```python
from build123d import *

# Parameters (mm, degrees)
SALIENTE_EXTRUIR1_DEPTH      = 6.5
SALIENTE_EXTRUIR1_DEPTH_BACK = 30
CROQUIS1_R                   = 2
CROQUIS2_W                   = 8
CROQUIS2_H                   = 10
CROQUIS2_H_2                 = 17.5
CORTAR_EXTRUIR2_DEPTH        = 20


with BuildPart() as part:
    # Croquis1 → Saliente-Extruir1 (new, two sides: drawn at the far end of the back side and taken through both)
    with BuildSketch(Plane.XY.offset(-SALIENTE_EXTRUIR1_DEPTH_BACK)):
        with BuildLine():
            Line((28.793175074, 33.764978898), (7.779852304, 40.592621349))
            Line((7.779852304, 40.592621349), (6.543784327, 36.788395284))
            ThreePointArc((6.543784327, 36.788395284), (4.366334456, 31.125676473), (9.776753104, 33.870679629))
            ThreePointArc((9.776753104, 33.870679629), (16.738586943, 32.414771462), (23.226590181, 29.500562652))
            ThreePointArc((23.226590181, 29.500562652), (25.990238441, 24.099644159), (27.557107096, 29.960752833))
            Line((27.557107096, 29.960752833), (28.793175074, 33.764978898))
        make_face()
        with Locations((6.543784327, 33.538395284)):
            Circle(CROQUIS1_R, mode=Mode.SUBTRACT)
        with Locations((25.646805026, 27.331447601)):
            Circle(CROQUIS1_R, mode=Mode.SUBTRACT)
    extrude(amount=SALIENTE_EXTRUIR1_DEPTH + SALIENTE_EXTRUIR1_DEPTH_BACK)

    # Croquis2 → Cortar-Extruir2 (cut)
    with BuildSketch(Plane(origin=(12.672781879, 39.002812158, 0), x_dir=(0.9510565162951536, -0.3090169943749473, 0), z_dir=(0.3090169943749473, 0.9510565162951536, 0))):
        with Locations((-3.390425382, 25)):
            Rectangle(CROQUIS2_W, CROQUIS2_H)
        with Locations((-3.390425382, -1.5)):
            Rectangle(CROQUIS2_W, CROQUIS2_H)
        with Locations((15.195679253, 11.75)):
            Rectangle(CROQUIS2_W, CROQUIS2_H_2)
    extrude(amount=-CORTAR_EXTRUIR2_DEPTH, mode=Mode.SUBTRACT)


solid = part.part
```
Part model, mm, in its own coordinate system. A direction names the side the tool comes from. Coordinates: 2 decimals unless noted, no trailing zeros. Order: outer loops, then holes, each group sorted by start corner. A loop starts at its lowest first (then second) coordinate and runs counter-clockwise, first axis right, second up. Notation, with made-up numbers: (-26, 39.25) -> (-1, 39.25) arc R25 cw to (-1, 67.25) -> close; hole circle Ø9 at (48.5, -0.5). An arc over 180 degrees is marked (long way). Put each result on its own line as item: value. Start each with the question number.
(1) Mould opens along Y. For faces 5 (the face through (12.424, 36.265, -24.93)), 6 (the face through (28.166, 31.836, 1.683)), 7 (the face through (26, 31, -20.5)) say: pulls with the +Y half, pulls with the -Y half, needs draft (parallel to the pull), parting line crosses it, or undercut.
(2) Band-saw the part on A-A (y = 26.5). Give the cut face in (x, z).
(3) Band-saw the part on C-C (y = 31). Give the cut face in (x, z).
(4) Band-saw the part on D-D (z = -8.5). Give the cut face in (x, y).
(5) Probe line 1 along Z through (x, y) = (27.5, 31.5); line 2 along X through (y, z) = (26, -2.5); line 3 along Z through (x, y) = (10.75, 39). List the from-to ranges inside material, lowest first. Write a range as [from, to].
(6) Which spindle directions (+Z, -Z, +X, -X, +Y, -Y) get a long thin tool onto all of the face, cutting with end or side? Do faces 1 (the face through (12.424, 36.265, 1.57)), 2 (the face through (28.166, 31.836, -25.316)), 3 (the face through (22.49, 32.99, -11.63)), 4 (the face through (22, 33, 6.5)). Say none if no direction does.
(7) Pin check, flat tips, straight feed: pin 1 Ø1.5 at (y, z) = (39, -2.5) entering from -X; pin 2 Ø5 at (x, y) = (8, 36.5) entering from +Z; pin 3 Ø3.5 at (x, y) = (25.65, 27.33) entering from -Z; pin 4 Ø10 at (x, z) = (10, 3) entering from -Y. Stop position of each tip, or through.
(8) Band-saw the part on B-B (x = 6). Give the cut face in (y, z).
Determined:
1. face 5: pulls with the +Y half
1. face 6: undercut
1. face 7: needs draft
2. outline: (22.5, -30) -> (23.83, -30) -> (23.83, -20.5) -> (22.5, -20.5) -> close; (22.5, -3) -> (23.83, -3) -> (23.83, 6.5) -> (22.5, 6.5) -> close; (27.47, -30) -> (28.79, -30) -> (28.79, -20.5) -> (27.47, -20.5) -> close; (27.47, -3) -> (28.79, -3) -> (28.79, 6.5) -> (27.47, 6.5) -> close
3. outline: (4.51, -20) -> (8.57, -20) -> (8.57, -3.5) -> (4.51, -3.5) -> close; (20.35, -30) -> (27.89, -30) -> (27.89, -20.5) -> (21.84, -20.5) -> (21.84, -3) -> (27.89, -3) -> (27.89, 6.5) -> (20.35, 6.5) -> close
4. outline: (6.54, 36.79) arc R3.25 ccw (long way) to (9.78, 33.87) arc R32.99 cw to (21.64, 30.37) -> (23.32, 35.54) -> (7.78, 40.59) -> close; hole circle Ø4 at (6.54, 33.54)
5. line 1: z = [-30, -20.5], [-3, 6.5]
5. line 2: x = [22.68, 24.15], [27.14, 28.61]
5. line 3: z = [-20, -3.5]
6. face 1: +Z, -X, +Y
6. face 2: +Z, -Z, +X
6. face 3: +X, -Y
6. face 4: +Z, +X, -X, +Y, -Y
7. pin 1: stops at x = 13.07
7. pin 2: stops at z = -3.5
7. pin 3: passes through
7. pin 4: stops at y = 32.93
8. outline: (30.33, -20) -> (31.61, -20) -> (31.61, -3.5) -> (30.33, -3.5) -> close; (35.46, -20) -> (36.74, -20) -> (36.74, -3.5) -> (35.46, -3.5) -> close
